Job drawing, mm, ordinate dimensions from the low corner. One solid piece. A direction names the side the tool comes from. Give positions to 0.01 mm unless a question says otherwise; leave off trailing zeros. Order: outer loops, then holes, each group sorted by start corner. A loop starts at its lowest first (then second) coordinate and runs counter-clockwise, first axis right, second up.
Item 1: Band-saw the part on A-A on x = 4.5. Give the cut face in (y, z), plus the area to 4 significant figures.
Item 2: Flat gauge pins, fed straight in: P1, Ø1, axis at y = 52, z = 6.5, coming from the -X side; P2, Ø3, axis at x = 7.5, y = 14, coming from the +Z side. Where does each tip first touch, or does it go through?
Item 3: Which spindle directions (+Z, -Z, +X, -X, +Y, -Y) get a long thin tool onto all of the face, cutting with end or side? Do the marked faces 1 and 2. Say none if no direction does.
Item 4: Band-saw the part on B-B on y = 7.5. Give the cut face in (x, z).
Item 5: Band-saw the part on C-C on z = 10.5. Give the cut face in (x, y).
Item 6: Wall check: L1, parallel to Z at x = 1.25, y = 23; L2, parallel to Y at x = 6.25, z = 9.75; L3, parallel to Y at x = 5.25, z = 11. Give the ranges that are in metal, low to high.
Item 7: Band-saw the part on D-D on y = 25. Give the cut face in (x, z).
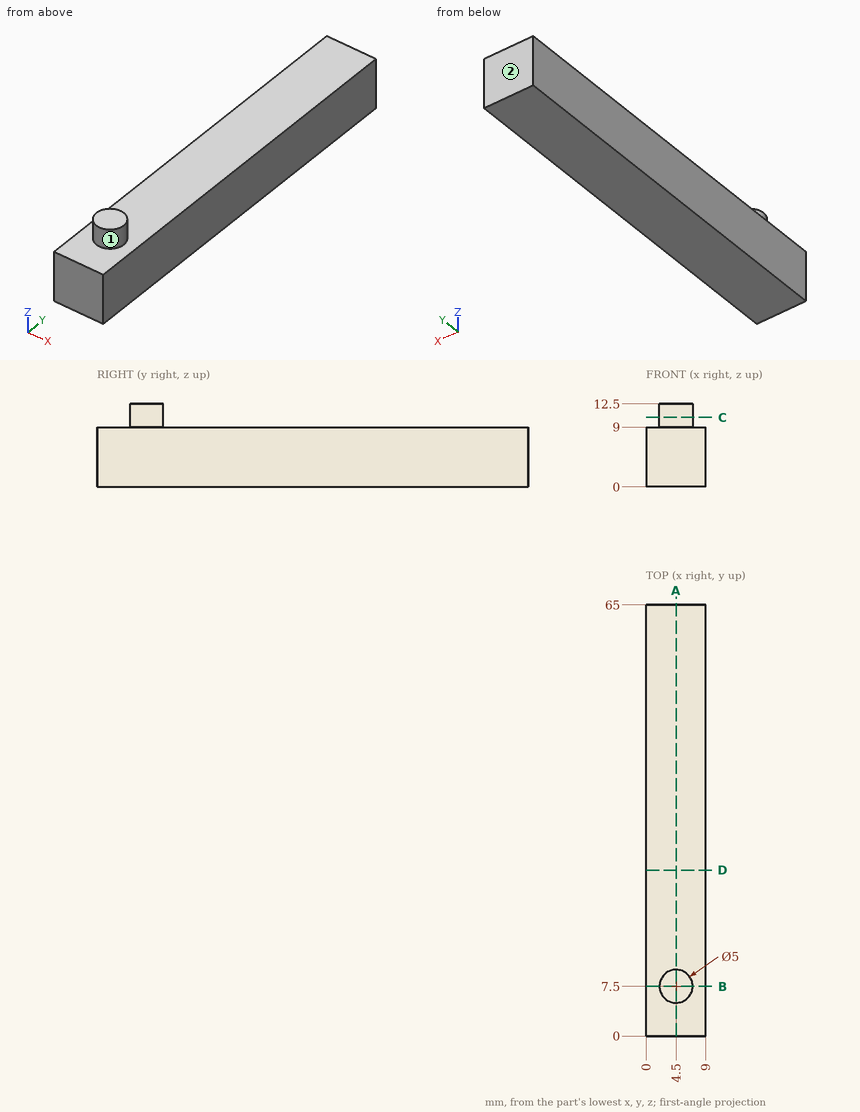
The answers:
1. outline: (0, 0) - (65, 0) - (65, 9) - (10, 9) - (10, 12.5) - (5, 12.5) - (5, 9) - (0, 9) - close
1. area: 602.5 mm2
2. P1: stops at x = 0
2. P2: stops at z = 9
3. face 1: +Z
3. face 2: +Z, -Z, +X, -X, +Y
4. outline: (0, 0) - (9, 0) - (9, 9) - (7, 9) - (7, 12.5) - (2, 12.5) - (2, 9) - (0, 9) - close
5. outline: circle Ø5 at (4.5, 7.5)
6. L1: z = 0 to 9
6. L2: y = 5.71 to 9.29
6. L3: y = 5.12 to 9.88
7. outline: (0, 0) - (9, 0) - (9, 9) - (0, 9) - close
